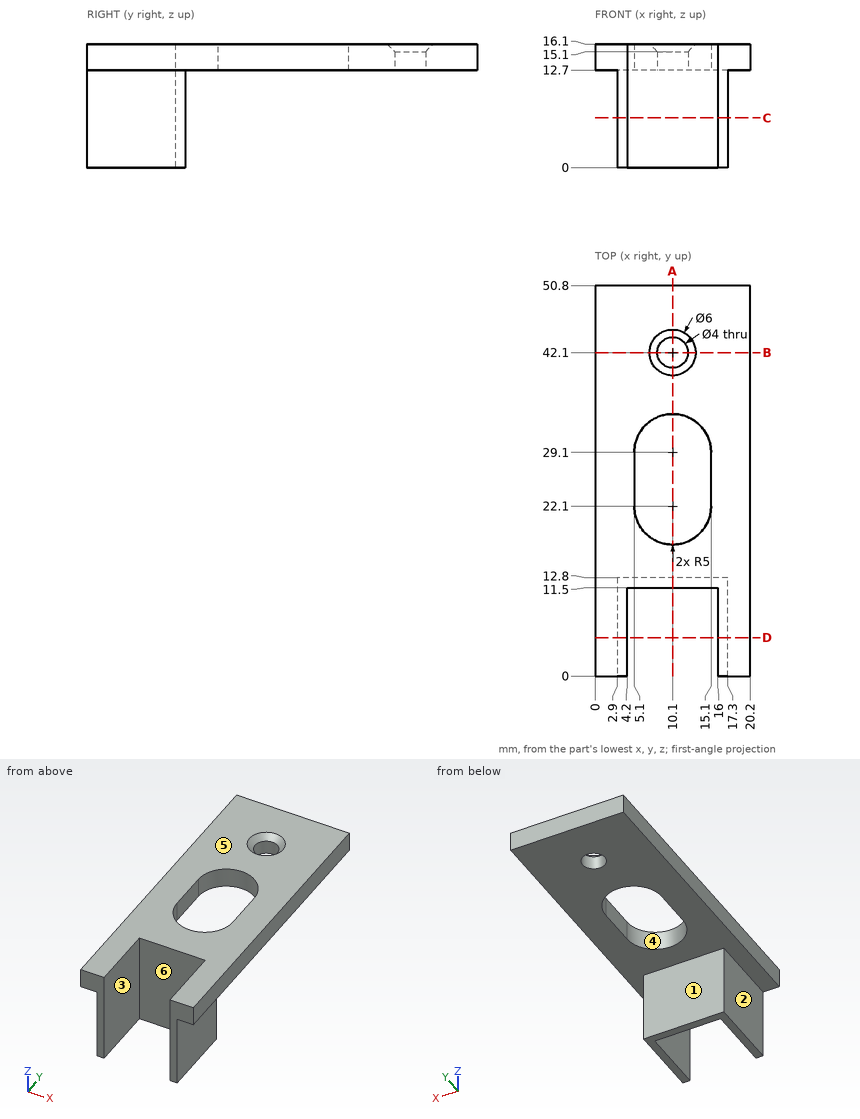
Part print with two shaded views. Sizes in mm from the minimum x, y, z corner. A direction names the side the tool comes from. Round coordinates to 2 decimals unless told otherwise and drop trailing zeros. Order: outer loops, then holes, each group sorted by start corner. A loop starts at its lowest first (then second) coordinate and runs counter-clockwise, first axis right, second up. Notation, with made-up numbers: M 35,72 L 71,72 A33 cw 71,108 Z; hole C 16.25,70.25 d6. An arc over 180 degrees is marked long. Use CSV: the item, a comma, the result in double quotes. Start each with the question number.
(1) Cut at C-C on z = 6.5. List the corners of the cut face in (x, y), then the cut area to 3 significant figures.
(2) Cut at A-A on x = 10.1. List the corners of the cut face in (y, z).
(3) Cut at D-D on y = 5. List the corners of the cut face in (x, z).
(4) Tool access for the marked faces 1, 2 and 3: list every direction of +Z, -Z, +X, -X, +Y, -Y with a clear straight run to the whole face (end or side of a thin tool).
(5) Mould opens along Y. For the marked faces 4, 5 and 6 say: +Y half, -Y half, draft (parallel to the pull), parting line (faces both ways), or undercut.
(6) Drill centre lines: probe 1 along Y at (x, z) = (10.1, 14.5); probe 2 along X at (y, z) = (5, 14.75); probe 3 along X at (y, z) = (42.1, 14.1). Where is each one in solid material? Low to high.
(7) Cut at B-B on y = 42.1. List the corners of the cut face in (x, z), then the cut area to 3 significant figures.
(8) Flat gauge pins, fed straight in: P1, Ø6, axis at x = 14, z = 4, coming from the +Y side; P2, Ø10, axis at x = 13, y = 22.5, coming from the -Z side; P3, Ø5, axis at y = 12, z = 6.5, coming from the +X side. Where does each tip first touch, or does it go through?
Findings:
1,outline,"M 2.9,0 L 4.2,0 L 4.2,11.5 L 16,11.5 L 16,0 L 17.3,0 L 17.3,12.8 L 2.9,12.8 Z"
1,area,"48.6 mm^2"
2,outline,"M 11.5,0 L 12.8,0 L 12.8,12.7 L 17.1,12.7 L 17.1,16.1 L 11.5,16.1 Z; M 34.1,12.7 L 40.1,12.7 L 40.1,15.1 L 39.1,16.1 L 34.1,16.1 Z; M 44.1,12.7 L 50.8,12.7 L 50.8,16.1 L 45.1,16.1 L 44.1,15.1 Z"
3,outline,"M 0,12.7 L 2.9,12.7 L 2.9,0 L 4.2,0 L 4.2,16.1 L 0,16.1 Z; M 16,0 L 17.3,0 L 17.3,12.7 L 20.2,12.7 L 20.2,16.1 L 16,16.1 Z"
4,face 1,"-Z, +X, -X, +Y"
4,face 2,"-Z, -X, +Y, -Y"
4,face 3,"+Z, -Z, -Y"
5,face 4,"undercut"
5,face 5,"draft"
5,face 6,"-Y half"
6,probe 1,"y = 11.5 to 17.1, 34.1 to 40.1, 44.1 to 50.8"
6,probe 2,"x = 0 to 4.2, 16 to 20.2"
6,probe 3,"x = 0 to 8.1, 12.1 to 20.2"
7,outline,"M 0,12.7 L 8.1,12.7 L 8.1,15.1 L 7.1,16.1 L 0,16.1 Z; M 12.1,12.7 L 20.2,12.7 L 20.2,16.1 L 13.1,16.1 L 12.1,15.1 Z"
7,area,"54.1 mm^2"
8,P1,"stops at y = 12.8"
8,P2,"stops at z = 12.7"
8,P3,"stops at x = 17.3"
